Model file for the job. Use its own axes, mm. A direction names the side the tool comes from. Round coordinates to 2 decimals unless told otherwise and drop trailing zeros. Loops run counter-clockwise (first coordinate to the right, second up) from the corner with the lowest first, then second, coordinate; pieces in that order, holes last.
from build123d import *

# Parameters (mm, degrees)
SKETCH1_R               = 30.48
BOSS_EXTRUDE1_DEPTH     = 25.4
SKETCH2_R               = 20.6502
CUT_EXTRUDE1_DEPTH      = 6.35
F_1_4_CLEARANCE_HOLE1_D = 6.5278


with BuildPart() as part:
    # Sketch1 → Boss-Extrude1 (new body)
    with BuildSketch(Plane(origin=(0, 0, 0), x_dir=(1, 0, 0), z_dir=(0, 1, 0))):
        with Locations(Location((0, 0, 0), (0, 0, 270))):
            Circle(SKETCH1_R)
    extrude(amount=BOSS_EXTRUDE1_DEPTH)

    # Sketch2 → Cut-Extrude1 (cut)
    with BuildSketch(Plane.XZ):
        with Locations(Location((0, 0, 0), (0, 0, 270))):
            Circle(SKETCH2_R)
    extrude(amount=-CUT_EXTRUDE1_DEPTH, mode=Mode.SUBTRACT)

    # Sketch4 → 3/4 NPT Tapped Hole1 (revolve, cut)
    with BuildSketch(Plane(origin=(0, 25.4, 0), x_dir=(0, 0, 1), z_dir=(1, 0, 0))):
        Polygon((0, 0), (0, 25.4), (11.5062, 25.4), (11.5062, 13.97), (12.914204892, 13.97), (13.3324854, 0), align=None)
    revolve(axis=Axis((0, 31.75, 0), (0, -1, 0)), mode=Mode.SUBTRACT)

    # 1/4 Clearance Hole1 (through all)
    with Locations(Plane(origin=(0, 25.4, 0), x_dir=(1, 0, 0), z_dir=(0, 1, 0))):
        with Locations((-24.636533331, 6.627886666), (-18.058184892, -18.021920393), (6.578348439, -24.649807059), (24.636533331, -6.627886666), (18.058184892, 18.021920393), (-6.578348439, 24.649807059)):
            Hole(F_1_4_CLEARANCE_HOLE1_D / 2)


solid = part.part
Q1. Slice it at B-B on x = 0. Give the cut face in (y, z).
Q2. Flat gauge pins, fed straight in: P1, Ø4, axis at x = -18.06, z = 18.02, coming from the -Y side; P2, Ø6, axis at y = 4, z = -10.5, coming from the +X side; P3, Ø2, axis at x = 20.5, y = 7, coming from the +Z side; P4, Ø8, axis at x = 14.5, y = 17.5, coming from the -Z side. Where does each tip first touch, or does it go through?
Q3. Slice it at C-C on y = 3.5. Give the cut face in (x, z).
Q4. Slice it at A-A on z = 0. Give the cut face in (x, y).
Q5. Slice it at D-D on z = -23. Give the cut face in (x, y), plus the area to 3 significant figures.
Q6. Tool access for faces 4 (the face through (7.987, 18.513, -10.417)), 5 (the face through (5.072, 12.522, 27.545)), 6 (the face through (-9, 6.35, -9)): list every direction of +Z, -Z, +X, -X, +Y, -Y with a clear straight run to the whole face (end or side of a thin tool).
Q7. Probe line 1 (X direction, y = 9.7, z = 0); line 2 (Z direction, x = -4, y = 22.75); line 3 (X direction, y = 18.5, z = -5). List the from-to ranges inside material, lowest first.
Q8. Pull direction X, two halves, no side cores. Call faces 1 (the face through (30.22, 12.52, -3.97)), 2 (the face through (-8.333, 12.522, -27.402)), 3 (the face through (0, 25.4, -14)): pulls with the +X half, pulls with the -X half, needs draft (parallel to the pull), parting line crosses it, or undercut.
Reply:
1. outline: (0, -30.48) - (25.4, -30.48) - (25.4, -13.33) - (11.43, -12.91) - (11.43, -11.51) - (6.35, -11.51) - (6.35, -20.65) - (0, -20.65) - close; (0, 20.65) - (6.35, 20.65) - (6.35, 11.51) - (11.43, 11.51) - (11.43, 12.91) - (25.4, 13.33) - (25.4, 30.48) - (0, 30.48) - close
2. P1: passes through
2. P2: stops at x = 29.54
2. P3: stops at z = 23.43
2. P4: stops at z = -28.61
3. outline: circle Ø60.96 at (0, 0); hole circle Ø6.53 at (-24.64, -6.63); hole circle Ø6.53 at (-18.06, 18.02); hole circle Ø41.3 at (0, 0); hole circle Ø6.53 at (-6.58, -24.65); hole circle Ø6.53 at (6.58, 24.65); hole circle Ø6.53 at (18.06, -18.02); hole circle Ø6.53 at (24.64, 6.63)
4. outline: (-30.48, 0) - (-20.65, 0) - (-20.65, 6.35) - (-11.51, 6.35) - (-11.51, 11.43) - (-12.91, 11.43) - (-13.33, 25.4) - (-30.48, 25.4) - close; (11.51, 6.35) - (20.65, 6.35) - (20.65, 0) - (30.48, 0) - (30.48, 25.4) - (13.33, 25.4) - (12.91, 11.43) - (11.51, 11.43) - close
5. outline: (-20, 0) - (-9.39, 0) - (-9.39, 25.4) - (-20, 25.4) - close; (-3.76, 0) - (20, 0) - (20, 25.4) - (-3.76, 25.4) - close
5. area: 873 mm2
6. face 4: +Y
6. face 5: +Y, -Y
6. face 6: -Y
7. line 1: x = -30.48 to -11.51, 11.51 to 30.48
7. line 2: z = -30.22 to -26.65, -22.65 to -12.64, 12.64 to 30.22
7. line 3: x = -30.07 to -27.47, -21.81 to -12.14, 12.14 to 30.07
8. face 1: parting line crosses it
8. face 2: undercut
8. face 3: needs draft
